Could you check a few things on this drawing? It's one solid part, dimensions in mm from its lowest x, y, z. A direction names the side the tool comes from. Round coordinates to 2 decimals unless told otherwise and drop trailing zeros. Write each loop counter-clockwise with the first axis right and the second up, starting at its lowest first coordinate (ties: lowest second). Pieces come first, ordered by that corner, then holes. Notation, with made-up numbers: (37.5, -35) -> (65.5, -35) arc R28 ccw to (65.5, -8) -> close; hole circle Ø2 at (-11.75, -34.75). An arc over 180 degrees is marked (long way). Return JSON: item names as keys, results as strings.
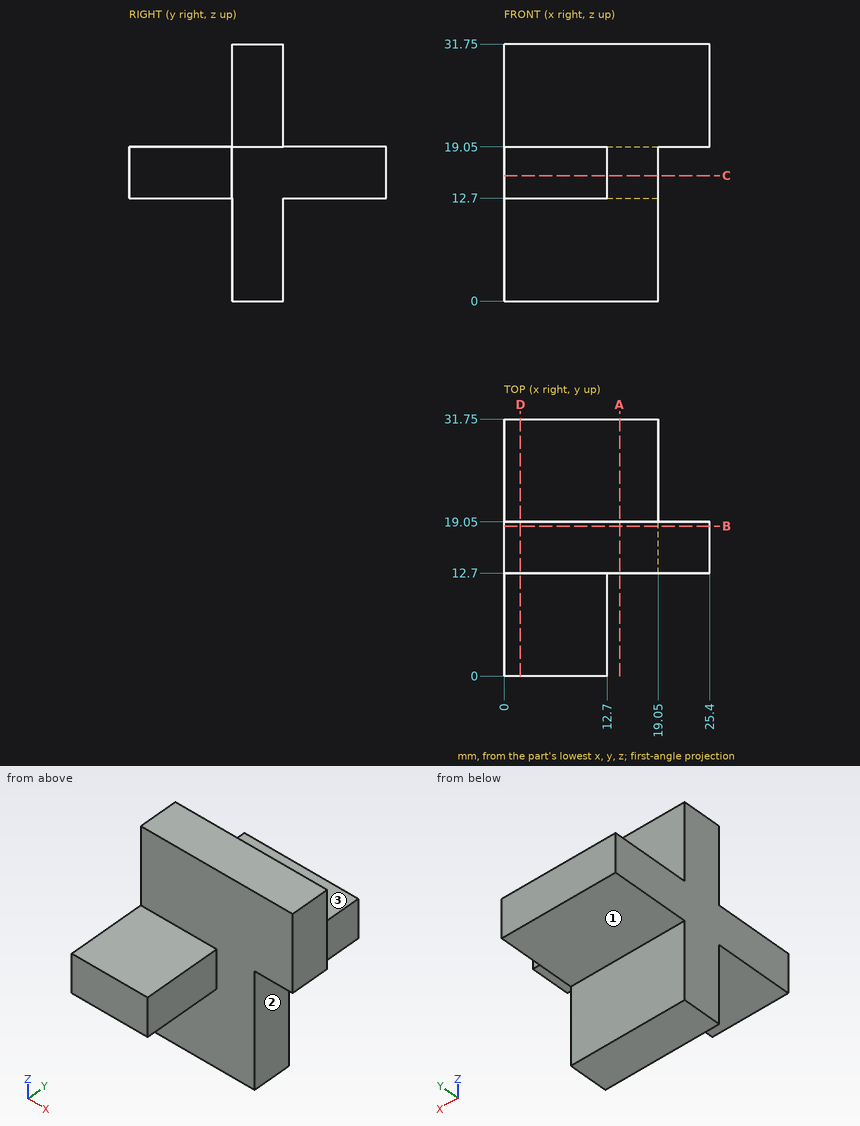
1) For the marked faces 1, 2 and 3, which set-ups out of +Z, -Z, +X, -X, +Y, -Y let a thin tool reach every point of the face, with its end or its side?
Return value:
{"face 1": "-Z, +X, -X, +Y", "face 2": "-Z, +X, +Y, -Y", "face 3": "+Z, +X, -X, +Y"}
2) I want a section at C-C, the plane z = 15.5. Please give me the cut outline in (x, y).
Return value:
{"outline": "(0, 0) -> (12.7, 0) -> (12.7, 12.7) -> (19.05, 12.7) -> (19.05, 31.75) -> (0, 31.75) -> close"}
3) If I drill on probe 1 along Z at (x, y) = (15.5, 24); probe 2 along X at (y, z) = (14, 6), over which ranges is the centre line in solid material (lowest first)? Write a range as [from, to].
Return value:
{"probe 1": "[12.7, 19.05]", "probe 2": "[0, 19.05]"}
4) I want a section at A-A, the plane x = 14.25. Please give me the cut outline in (y, z).
Return value:
{"outline": "(12.7, 0) -> (19.05, 0) -> (19.05, 12.7) -> (31.75, 12.7) -> (31.75, 19.05) -> (19.05, 19.05) -> (19.05, 31.75) -> (12.7, 31.75) -> close"}
5) I want a section at B-B, the plane y = 18.5. Please give me the cut outline in (x, z), and give its area (3 significant figures).
Return value:
{"outline": "(0, 0) -> (19.05, 0) -> (19.05, 19.05) -> (25.4, 19.05) -> (25.4, 31.75) -> (0, 31.75) -> close", "area": "685 mm²"}
6) Will these pins go through, and if not, where does the flat tip stop? pin 1 Ø1.9 at (x, y) = (21.5, 15) entering from -Z; pin 2 Ø2 at (x, z) = (3, 7.5) entering from -Y; pin 3 Ø6.5 at (x, y) = (5.5, 8.5) entering from +Z.
Return value:
{"pin 1": "z = 19.05", "pin 2": "y = 12.7", "pin 3": "z = 19.05"}
7) I want a section at D-D, the plane x = 2. Please give me the cut outline in (y, z), and give its area (3 significant figures).
Return value:
{"outline": "(0, 12.7) -> (12.7, 12.7) -> (12.7, 0) -> (19.05, 0) -> (19.05, 12.7) -> (31.75, 12.7) -> (31.75, 19.05) -> (19.05, 19.05) -> (19.05, 31.75) -> (12.7, 31.75) -> (12.7, 19.05) -> (0, 19.05) -> close", "area": "363 mm²"}
